Can you work these out from the model? Positions are in its coordinate system, mm. A direction names the side the tool comes from. Give positions to 0.01 mm unless a question says otherwise; leave off trailing zeros. Write each loop counter-clockwise with the first axis right and the second up, starting at its lowest first coordinate (ties: lowest second). Pieces come first, ordered by that corner, then holes. Notation, with made-up numbers: (41.5, 70.25) -> (52.5, 70.25) arc R12 cw to (52.5, 76.25) -> close; hole circle Ø5 at (-11.5, 57). An arc over 180 degrees is marked (long way). One line per item, written item: value.
Autodesk Fusion 360 part; units mm, degrees
sketch "Sketch1" plane through (0, 0, 0) normal (0, 0, 1) x (1, 0, 0)
  line L0 (0, 0) -> (100, 0) construction
  line L1 (0, 0) -> (-100, 0) construction
  line L2 (0, -3) -> (100, -3) construction
  line L3 (0, -3) -> (-100, -3) construction
  circle A0 centre (0, 0) radius 24.6 construction
  circle A1 centre (0, 0) radius 28.5 construction
  line L4 (0, -23) -> (100, -23) construction
  line L5 (0, -23) -> (-100, -23) construction
  line L6 (0, 0) -> (0, -150) construction
  line L7 (0, 0) -> (0, 150) construction
  line L8 (-30.5, 0) -> (-30.5, -150) construction
  line L9 (-30.5, 0) -> (-30.5, 150) construction
  line L10 (30.5, 0) -> (30.5, 150) construction
  line L11 (30.5, 0) -> (30.5, -150) construction
  line L12 (-30.5, -23) -> (-42.5, -23)
  line L13 (-42.5, -23) -> (-42.5, -18)
  line L14 (-42.5, -18) -> (-12.5, -18) construction
  line L15 (-42.5, -18) -> (-27.5, -3)
  line L16 (-24.5998, -0.0998) -> (-24.5, 0)
  line L17 (-24.4164, -3) -> (-27.5, -3)
  line L18 (24.4164, -3) -> (27.5, -3)
  line L19 (42.5, -18) -> (27.5, -3)
  line L20 (30.5, -23) -> (42.5, -23)
  line L21 (42.5, -23) -> (42.5, -18)
  arc A2 (-24.4164, -3) -> (24.4164, -3) centre (0, 0) ccw
  line L22 (0, -45) -> (-100, -45) construction
  line L23 (0, -45) -> (100, -45) construction
  circle A3 centre (0, -45) radius 6
  circle A4 centre (0, -45) radius 12.5 construction
  line L24 (-12.5, -45) -> (-12.5, -29)
  line L25 (-30.5, -23) -> (-18.5, -23)
  line L26 (12.5, -45) -> (12.5, -29)
  line L27 (30.5, -23) -> (18.5, -23)
  arc A5 (-12.5, -45) -> (12.5, -45) centre (0, -45) ccw
  arc A6 (-12.5, -29) -> (-18.5, -23) centre (-18.5, -29) ccw
  arc A7 (18.5, -23) -> (12.5, -29) centre (18.5, -29) ccw
  dimension "d4" = 3
  dimension "d5" = 49.2
  dimension "d6" = 57
  dimension "d7" = 23
  dimension "d10" = 30.5
  dimension "d11" = 30.5
  dimension "d12" = 12
  dimension "d13" = 5
  dimension "d14" = 45
  dimension "d16" = 24.6
  dimension "d17" = 45
  dimension "d18" = 12
  dimension "d19" = 25
  dimension "d20" = 6
  dimension "d21" = 6
extrude "Extrude1" add sketch "Sketch1" along normal mid plane 42
sketch "Sketch2" plane through (0, 0, 0) normal (0, 1, 0) x (1, 0, 0)
  line L0 (-24.4164, 21) -> (24.4164, 21) construction
  line L1 (-27.5, 21) -> (-24.4164, 21) construction
  line L2 (-42.5, 21) -> (-27.5, 21) construction
  line L3 (24.4164, 21) -> (27.5, 21) construction
  line L4 (27.5, 21) -> (42.5, 21) construction
  line L5 (6, -21) -> (-6, -21) construction
  line L6 (18.5, -21) -> (42.5, -21) construction
  line L7 (42.5, -21) -> (27.5, -21) construction
  line L8 (27.5, -21) -> (24.4164, -21) construction
  line L9 (24.4164, -21) -> (-24.4164, -21) construction
  line L10 (-24.4164, -21) -> (-27.5, -21) construction
  line L11 (-27.5, -21) -> (-42.5, -21) construction
  line L12 (-42.5, -21) -> (-18.5, -21) construction
  line L13 (-12.5, -21) -> (-18.5, -21) construction
  line L14 (-12.5, -21) -> (12.5, -21) construction
  line L15 (18.5, -21) -> (12.5, -21) construction
  line L16 (42.5, 21) -> (42.5, -21) construction
  line L17 (42.5, -21) -> (42.5, 21) construction
  line L18 (-42.5, 21) -> (-42.5, -21) construction
  line L19 (-42.5, -21) -> (-42.5, 21) construction
  circle A0 centre (-30.5, 0) radius 12 construction
  circle A1 centre (30.5, 0) radius 12 construction
  line L20 (0, 21) -> (0, -21) construction
  line L21 (-12.5, 21) -> (-12.5, -21) construction
  line L22 (12.5, 21) -> (12.5, -21) construction
  line L23 (-12.5, 21) -> (12.5, 21)
  line L24 (-12.5, -21) -> (12.5, -21)
  line L25 (12.5, -21) -> (35.3207, -10.9891)
  line L26 (12.5, 21) -> (35.3207, 10.9891)
  line L27 (-12.5, 21) -> (-35.3207, 10.9891)
  line L28 (-12.5, -21) -> (-35.3207, -10.9891)
  arc A2 (35.3207, -10.9891) -> (35.3207, 10.9891) centre (30.5, 0) ccw
  arc A3 (-35.3207, 10.9891) -> (-35.3207, -10.9891) centre (-30.5, 0) ccw
  line L29 (12.5, 21) -> (42.5, 21)
  line L30 (12.5, -21) -> (42.5, -21)
  line L31 (42.5, -21) -> (42.5, 21)
  line L32 (-42.5, 21) -> (-12.5, 21)
  line L33 (-42.5, -21) -> (-12.5, -21)
  line L34 (-42.5, -21) -> (-42.5, 21)
  circle A4 centre (30.5, 0) radius 6
  circle A5 centre (-30.5, 0) radius 6
  dimension "d24" = 24
  dimension "d25" = 24
  dimension "d26" = 12.5
  dimension "d27" = 12.5
  dimension "d28" = 12
  dimension "d29" = 12
extrude "Extrude2" cut sketch "Sketch2" against normal through all contours L27 A3 L32 L34 | L26 A2 L29 L31 | L28 A3 L33 L34 | L25 A2 L30 L31 | A4 | A5
sketch "Sketch3" plane through (0, 0, 0) normal (1, 0, 0) x (0, 0, -1)
  line L0 (-21, -51) -> (-21, -39) construction
  line L1 (-21, -29) -> (-21, -21.1875) construction
  line L2 (-21, -24.6) -> (-21, -21.1875) construction
  line L3 (-21, -21.1875) -> (-21, -29) construction
  line L4 (-21, -29) -> (-21, -45) construction
  line L5 (-21, -45) -> (-21, -57.5) construction
  line L6 (-21, -45) -> (-21, -29) construction
  line L7 (21, -21.1875) -> (21, -29) construction
  line L8 (21, -29) -> (21, -45) construction
  line L9 (21, -57.5) -> (21, -45) construction
  line L10 (21, -45) -> (21, -29) construction
  line L11 (21, -29) -> (21, -21.1875) construction
  line L12 (21, -21.1875) -> (21, -24.6) construction
  line L13 (21, -39) -> (21, -51) construction
  line L14 (21, -45) -> (-21, -45) construction
  line L15 (-21, -45) -> (-21, -57.5) construction
  line L16 (-21, -45) -> (21, -45) construction
  line L17 (21, -57.5) -> (21, -45) construction
  line L18 (21, -45) -> (-21, -45) construction
  line L19 (-21, -45) -> (-21, -29) construction
  line L20 (-21, -29) -> (21, -29) construction
  line L21 (21, -29) -> (21, -45) construction
  line L22 (-5.1962, -3) -> (-14.4199, -3) construction
  line L23 (14.4199, -3) -> (5.1962, -3) construction
  line L24 (-5.1962, -3) -> (5.1962, -3) construction
  arc A0 (-5.1962, -3) -> (5.1962, -3) centre (0, -6) ccw construction
  line L25 (-5.1962, -3) -> (5.1962, -3) construction
  line L26 (6, -23) -> (-6, -23) construction
  line L27 (0, 0) -> (0, -75) construction
  line L28 (-6, 0) -> (-6, -75) construction
  line L29 (-8, 0) -> (-8, -75) construction
  line L30 (6, 0) -> (6, -75) construction
  line L31 (8, 0) -> (8, -75) construction
  line L32 (21, -57.5) -> (-21, -57.5) construction
  line L33 (21, -57.5) -> (15, -57.5)
  line L34 (-21, -57.5) -> (-15, -57.5)
  line L35 (0, 0) -> (40, 0) construction
  line L36 (0, 0) -> (-40, 0) construction
  line L37 (0, -28.5) -> (-40, -28.5) construction
  line L38 (15, -57.5) -> (15, -32)
  line L39 (-15, -57.5) -> (-15, -32)
  line L40 (-12, -29) -> (12, -29)
  line L41 (15, -57.5) -> (-15, -57.5)
  arc A1 (15, -32) -> (12, -29) centre (12, -32) ccw
  arc A2 (-12, -29) -> (-15, -32) centre (-12, -32) ccw
  line L42 (0, -3) -> (-8, -3)
  line L43 (0, -3) -> (8, -3)
  line L44 (14.4199, -14) -> (5.1962, -14) construction
  line L45 (-5.1962, -14) -> (5.1962, -14) construction
  line L46 (-5.1962, -14) -> (-14.4199, -14) construction
  line L47 (6, -14) -> (8, -3)
  line L48 (-6, -14) -> (-8, -3)
  line L49 (-6, -14) -> (6, -14)
  point P0 (-15.7726, -3)
  point P1 (15.7726, -3)
  point P2 (21, -21.1875)
  point P3 (-21, -21.1875)
  dimension "d32" = 6
  dimension "d33" = 8
  dimension "d34" = 6
  dimension "d35" = 8
  dimension "d36" = 6
  dimension "d37" = 6
  dimension "d41" = 3
  dimension "d42" = 3
  dimension "d43" = 8
  dimension "d44" = 11
extrude "Extrude3" cut sketch "Sketch3" along normal through all and the other way through all
equation "d5 = ( 24.6 * 2 ) * 1 mm"
equation "d6 = ( 28.5 * 2 ) * 1 mm"
1) We'd pull the mould along Z, two halves only. Please class faces 4 (the face through (-42.5, -19.5, -0.2)), 5 (the face through (26.29, -15.82, 14.95)), 6 (the face through (23, -14, 0)): released by +Z, released by -Z, zero draft, split by the parting line, or undercut.
Answer list:
face 4: split by the parting line
face 5: released by +Z
face 6: undercut
2) If we section it at B-B (y = -33.5): Write out the boundary of the cut face in (x, z).
Answer list:
outline: (-12.5, -21) -> (12.5, -21) -> (12.5, -15) -> (-12.5, -15) -> close; (-12.5, 15) -> (12.5, 15) -> (12.5, 21) -> (-12.5, 21) -> close
3) If we section it at C-C (z = 0): Write out the boundary of the cut face in (x, y), and give its area (3 significant figures).
Answer list:
outline: (-42.5, -23) -> (-36.5, -23) -> (-36.5, -14) -> (-38.5, -14) -> (-42.5, -18) -> close; (-24.5, -23) -> (-18.5, -23) arc R6 cw to (-12.5, -29) -> (12.5, -29) arc R6 cw to (18.5, -23) -> (24.5, -23) -> (24.5, -14) -> (20.23, -14) arc R24.6 cw to (-20.23, -14) -> (-24.5, -14) -> close; (36.5, -23) -> (42.5, -23) -> (42.5, -18) -> (38.5, -14) -> (36.5, -14) -> close
area: 397 mm^2
4) If we section it at D-D (y = -44): Write out the boundary of the cut face in (x, z), and give its area (3 significant figures).
Answer list:
outline: (-12.5, -21) -> (-5.92, -21) -> (-5.92, -15) -> (-12.5, -15) -> close; (-12.5, 15) -> (-5.92, 15) -> (-5.92, 21) -> (-12.5, 21) -> close; (5.92, -21) -> (12.5, -21) -> (12.5, -15) -> (5.92, -15) -> close; (5.92, 15) -> (12.5, 15) -> (12.5, 21) -> (5.92, 21) -> close
area: 158 mm^2
5) I need wall thicknesses on L1, parallel to X at y = -45, z = 17.85; L2, parallel to Y at x = 0, z = -18.05; L3, parallel to X at y = -18.75, z = 0. Which ranges of each line are inside material? Lowest first, please.
Answer list:
L1: x = -12.5 to -6, 6 to 12.5
L2: y = -57.5 to -51, -39 to -24.6
L3: x = -42.5 to -36.5, -24.5 to -15.92, 15.92 to 24.5, 36.5 to 42.5
6) If we section it at A-A (x = 0): Write out the boundary of the cut face in (y, z).
Answer list:
outline: (-57.5, -21) -> (-51, -21) -> (-51, -15) -> (-57.5, -15) -> close; (-57.5, 15) -> (-51, 15) -> (-51, 21) -> (-57.5, 21) -> close; (-39, -21) -> (-24.6, -21) -> (-24.6, 21) -> (-39, 21) -> (-39, 15) -> (-32, 15) arc R3 cw to (-29, 12) -> (-29, -12) arc R3 cw to (-32, -15) -> (-39, -15) -> close
7) For faces 1 (the face through (37, -14, 0)), 2 (the face through (3, -39, -15)), 3 (the face through (-36.494, -18.437, -0.264)), which set-ups out of +Z, -Z, +X, -X, +Y, -Y let a thin tool reach every point of the face, with its end or its side?
Answer list:
face 1: +X, -X, +Y
face 2: +X, -X, -Y
face 3: +Y, -Y
8) Will these pins go through, and if not, where does the flat tip stop? pin 1 (2.5 mm diameter, centred on y = -36.5, z = 18.5, fed in from -X); pin 2 (11 mm diameter, centred on x = -30.5, z = 0, fed in from +Y); pin 3 (5 mm diameter, centred on y = -19, z = -11.5, fed in from -X); pin 4 (4 mm diameter, centred on x = -17, z = -14.5, fed in from -Y).
Answer list:
pin 1: stops at x = -12.5
pin 2: passes through
pin 3: stops at x = -38.44
pin 4: stops at y = -24.13
